The model under review builds one solid part; all positions refer to its coordinate system, in mm. Face numbers are marked on the shaded views. Coordinates: 2 decimals unless noted, no trailing zeros. Write each loop counter-clockwise with the first axis right and the second up, starting at its lowest first coordinate (ties: lowest second). Pieces come first, ordered by that corner, then holes.
1) Add section A-A, the plane z = 121. Give the number of separate pieces and of enclosed holes in the cut face, then the cut area to 3 significant figures.
2) For line 1 (X direction, y = -94.25, z = 123); line 2 (Z direction, x = -37, y = -106.25); line 3 (Y direction, x = -75.5, z = 135.8), list the stretches that pass through material, from the lowest coordinate up.
3) Mouldability with a two-part tool opening along X and no side actions: class the marked faces 1, 2 and 3 as released by +X, released by -X, zero draft, split by the parting line, or undercut.
4) Add section C-C, the plane z = 184.5. State the section outline as (x, y) points.
5) Add section D-D, the plane y = -93.5. State the section outline as (x, z) points.
6) Add section B-B, the plane x = -36.5. State the section outline as (y, z) points.
7) For P1, Ø15, axis at x = -45.75, y = -102.8, coming from the +Z side; P2, Ø3.5, axis at x = -8.51, z = 121.53, coming from the -Y side; P3, Ø6, axis at x = -72.5, y = -113, coming from the -Z side; P4, Ø1.5, axis at x = -49.5, z = 207.5, coming from the -Y side, all flat-tipped, find the tip position at first contact; note any pin that passes through.
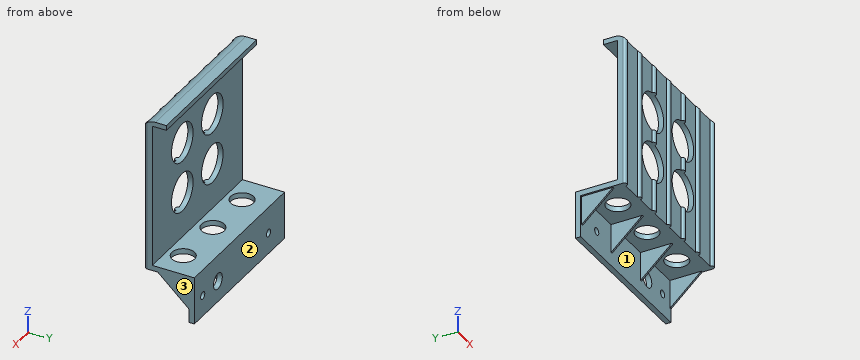
from build123d import *

# Parameters (mm, degrees)
BOSS_EXTRU_1_DEPTH           = 92
NERVURE2_REACH               = 267.583
ESQUISSE3_WALL_W             = 557.337159988
ESQUISSE3_WALL_H             = 1
R_P_TITION_LIN_AIRE1_COUNT   = 4
R_P_TITION_LIN_AIRE1_PITCH   = 30
ESQUISSE4_R                  = 6.5
ENL_V_MAT_EXTRU_1_DEPTH      = 3
ESQUISSE6_R                  = 1.5
BOSS_EXTRU_2_DEPTH           = 87.544216856
R_P_TITION_LIN_AIRE2_COUNT   = 7
R_P_TITION_LIN_AIRE2_PITCH   = 14.833333333
ENL_V_MAT_EXTRU_2_DEPTH      = 3
ENL_V_MAT_EXTRU_2_DEPTH_BACK = 3
ESQUISSE5_R                  = 11
ENL_V_START                  = -92
ENL_V_MAT_EXTRU_3_DEPTH      = 92
CONG_1_R                     = 8
ESQUISSE9_R                  = 4.5
ENL_V_MAT_EXTRU_5_DEPTH      = 3
ESQUISSE8_R                  = 2.1
ENL_V_MAT_EXTRU_4_DEPTH      = 3


with BuildPart() as part:
    # Esquisse1 → Boss.-Extru.1 (new body)
    with BuildSketch(Plane(origin=(0, 0, 0), x_dir=(0, 0, -1), z_dir=(1, 0, 0))):
        Polygon((-109.489716306, -87.800176517), (-136.569905432, -87.800176517), (-136.569905432, -111.800176517), (-218.114122288, -111.800176517), (-218.314122288, -111.800176517), (-218.314122288, -103.710391053), (-221.114122288, -103.710391053), (-221.114122288, -114.800176517), (-133.569905432, -114.800176517), (-133.569905432, -90.800176517), (-109.489716306, -90.800176517), align=None)
    extrude(amount=-BOSS_EXTRU_1_DEPTH)

    # Esquisse3 wall → Nervure2 (add, up to next)
    with BuildSketch(Plane(origin=(0, -99.717919792, 125.413574296), x_dir=(0, -0.737906584765, 0.674902861278), z_dir=(0, -0.674902861278, -0.737906584765)), mode=Mode.PRIVATE) as nervure2_sk1:
        with Locations((0, 0.5)):
            Rectangle(ESQUISSE3_WALL_W, ESQUISSE3_WALL_H)
    nervure2_tool1 = extrude(nervure2_sk1.sketch, amount=-NERVURE2_REACH, mode=Mode.PRIVATE) - part.part
    nervure2 = nervure2_tool1.solids().sort_by_distance((0, -99.717919792, 125.413574296))[0]
    add(nervure2)

    # Répétition linéaire1: Nervure2 ×4
    with Locations(*[(-i * R_P_TITION_LIN_AIRE1_PITCH, 0, 0) for i in range(1, R_P_TITION_LIN_AIRE1_COUNT)]):
        add(nervure2)

    # Esquisse4 → Enlèv. mat.-Extru.1 (cut)
    with BuildSketch(Plane(origin=(0, 0, 133.569905432), x_dir=(-1, 0, 0), z_dir=(0, 0, -1))):
        with Locations((15.5, -102.800176517)):
            Circle(ESQUISSE4_R)
        with Locations((45.75, -102.800176517)):
            Circle(ESQUISSE4_R)
        with Locations((75.5, -102.800176517)):
            Circle(ESQUISSE4_R)
    extrude(amount=-ENL_V_MAT_EXTRU_1_DEPTH, mode=Mode.SUBTRACT)

    # Esquisse6 → Boss.-Extru.2 (add)
    with BuildSketch(Plane(origin=(0, 0, 133.569905432), x_dir=(-1, 0, 0), z_dir=(0, 0, -1))):
        with Locations((1.5, -114.800176517)):
            Circle(ESQUISSE6_R)
    boss_extru_2 = extrude(amount=-BOSS_EXTRU_2_DEPTH)

    # Répétition linéaire2: Boss.-Extru.2 ×7
    with Locations(*[(-i * R_P_TITION_LIN_AIRE2_PITCH, 0, 0) for i in range(1, R_P_TITION_LIN_AIRE2_COUNT)]):
        add(boss_extru_2)

    # Esquisse5 → Enlèv. mat.-Extru.2 (cut, two sides: drawn at the far end of the back side and taken through both)
    with BuildSketch(Plane(origin=(0, -114.800176517, 0), x_dir=(-1, 0, 0), z_dir=(0, -1, 0)).offset(-ENL_V_MAT_EXTRU_2_DEPTH_BACK)):
        with Locations(Location((30.666666667, -162.751311051, 0), (0, 0, 264.78409143))):
            Circle(ESQUISSE5_R)
        with Locations(Location((61.333333333, -162.751311051, 0), (0, 0, 275.21590857))):
            Circle(ESQUISSE5_R)
        with Locations(Location((61.333333333, -191.93271667, 0), (0, 0, 275.21590857))):
            Circle(ESQUISSE5_R)
        with Locations(Location((30.666666667, -191.93271667, 0), (0, 0, 264.78409143))):
            Circle(ESQUISSE5_R)
    extrude(amount=ENL_V_MAT_EXTRU_2_DEPTH + ENL_V_MAT_EXTRU_2_DEPTH_BACK, mode=Mode.SUBTRACT)

    # Esquisse7 → Enlèv. mat.-Extru.3 (cut)
    with BuildSketch(Plane(origin=(0, 0, 0), x_dir=(0, 0, -1), z_dir=(1, 0, 0)).offset(ENL_V_START)):
        Polygon((-221.114122288, -113.242817204), (-218.056762976, -116.300176517), (-221.114122288, -116.300176517), align=None)
    extrude(amount=ENL_V_MAT_EXTRU_3_DEPTH, mode=Mode.SUBTRACT)

    # Congé1
    # the kernel refuses this fillet: 8 mm, written as the material it takes off along each edge
    with BuildSketch(Plane(origin=(-100.284271247, -113.242817204, 221.114122288), x_dir=(0, -0.7071067811865497, -0.7071067811865454), z_dir=(1, 0, 0))) as cong_1_piece_1:
        with BuildLine():
            CenterArc((CONG_1_R * 0.414213562373, CONG_1_R), CONG_1_R, 225, 45)
            Line((-CONG_1_R * 0.292893218813, CONG_1_R * 0.292893218813), (0, 0))
            Line((0, 0), (CONG_1_R * 0.414213562373, 0))
        make_face()
    extrude(amount=108.568542495, mode=Mode.SUBTRACT)

    # Esquisse9 → Enlèv. mat.-Extru.5 (cut)
    with BuildSketch(Plane.XZ.offset(90.800176517)):
        with Locations(Location((-24, 121.529810869, 0), (0, 0, 270))):
            Circle(ESQUISSE9_R)
    extrude(amount=-ENL_V_MAT_EXTRU_5_DEPTH, mode=Mode.SUBTRACT)

    # Esquisse8 → Enlèv. mat.-Extru.4 (cut)
    with BuildSketch(Plane.XZ.offset(90.800176517)):
        with Locations(Location((-8.506517848, 121.529810869, 0), (0, 0, 270))):
            Circle(ESQUISSE8_R)
        with Locations(Location((-75.666666667, 121.529810869, 0), (0, 0, 270))):
            Circle(ESQUISSE8_R)
    extrude(amount=-ENL_V_MAT_EXTRU_4_DEPTH, mode=Mode.SUBTRACT)


solid = part.part
Geometry results:
1. separate pieces: 4
1. enclosed holes: 0
1. area: 241 mm2
2. line 1: x = -91 to -90, -61 to -60, -31 to -30, -1 to 0
2. line 2: z = 133.57 to 136.57, 218.31 to 221.11
2. line 3: y = -116.29 to -109.3, -96.3 to -87.8
3. face 1: undercut
3. face 2: zero draft
3. face 3: released by +X
4. outline: (-92, -114.8) arc R1.5 ccw to (-89, -114.8) - (-77.17, -114.8) arc R1.5 ccw to (-74.17, -114.8) - (-69.44, -114.8) - (-69.44, -111.8) - (-92, -111.8) - close; (-53.22, -114.8) - (-47.5, -114.8) arc R1.5 ccw to (-44.5, -114.8) - (-38.78, -114.8) - (-38.78, -111.8) - (-53.22, -111.8) - close; (-22.56, -114.8) - (-17.83, -114.8) arc R1.5 ccw to (-14.83, -114.8) - (-3, -114.8) arc R1.5 ccw to (0, -114.8) - (0, -111.8) - (-22.56, -111.8) - close
5. outline: (-92, 133.57) - (-91, 133.57) - (-91, 119.73) - (-90, 119.73) - (-90, 133.57) - (-61, 133.57) - (-61, 119.73) - (-60, 119.73) - (-60, 133.57) - (-31, 133.57) - (-31, 119.73) - (-30, 119.73) - (-30, 133.57) - (-1, 133.57) - (-1, 119.73) - (0, 119.73) - (0, 136.57) - (-92, 136.57) - close
6. outline: (-114.8, 133.57) - (-90.8, 133.57) - (-90.8, 109.49) - (-87.8, 109.49) - (-87.8, 136.57) - (-111.8, 136.57) - (-111.8, 153.43) - (-114.8, 153.43) - close; (-114.8, 172.08) - (-111.8, 172.08) - (-111.8, 182.61) - (-114.8, 182.61) - close; (-114.8, 201.26) - (-111.8, 201.26) - (-111.8, 218.31) - (-103.71, 218.31) - (-103.71, 221.11) - (-109.93, 221.11) arc R8 ccw to (-114.8, 219.46) - close
7. P1: stops at z = 221.11
7. P2: passes through
7. P3: stops at z = 133.57
7. P4: stops at y = -114.8
